The listing builds one solid part. Answer for the finished solid, in the listing's coordinates (mm). A direction names the side the tool comes from. Coordinates: 2 decimals unless noted, no trailing zeros. Write each loop counter-clockwise with the first axis right and the second up, starting at its lowest first coordinate (ties: lowest second). Pieces come first, ordered by that corner, then holes. Notation, with made-up numbers: M 27.25,-32 L 76.25,-32 A13 cw 76.25,-18 Z; hole C 7,83 d8. An arc over 180 degrees is marked long. Put each result on its own line as item: value. Start each with the question number.
Autodesk Fusion 360 part; units mm, degrees
sketch "Sketch1" plane through (0, 0, 0) normal (1, 0, 0) x (0, 1, 0)
  line L0 (-95, 52.5) -> (95, 52.5)
  line L1 (95, 52.5) -> (95, -52.5)
  line L2 (95, -52.5) -> (-95, -52.5)
  line L3 (-95, -52.5) -> (-95, 52.5)
  line L4 (95, 52.5) -> (-95, -52.5) construction
  line L5 (-95, 52.5) -> (95, -52.5) construction
  line L6 (92, -49.5) -> (-92, -49.5)
  line L7 (-92, -49.5) -> (-92, 49.5)
  line L8 (-92, 49.5) -> (92, 49.5)
  line L9 (92, 49.5) -> (92, -49.5)
  dimension "d1" = 190
  dimension "d2" = 105
  dimension "d5" = 3
extrude "Extrude1" add sketch "Sketch1" along normal blind 14 contours L0 L1 L2 L3 | L6 L7 L8 L9
extrude "Extrude2" cut sketch "Sketch1" along normal blind 10 contours L6 L7 L8 L9
fillet "Fillet1" radius 2.5 4 edges at (14, 0, -52.5) (14, 95, 0) (14, 0, 52.5) (14, -95, 0)
sketch "Sketch2" plane through (14, 0, 0) normal (1, 0, 0) x (0, 1, 0)
  line L0 (92.5, 50) -> (-92.5, 50)
  line L1 (-92.5, 50) -> (-92.5, -50)
  line L2 (-92.5, -50) -> (92.5, -50)
  line L3 (92.5, -50) -> (92.5, 50)
  circle A0 centre (0, 0) radius 7.5
  dimension "d10" = 15
extrude "Extrude3" cut sketch "Sketch2" against normal blind 40 contours A0
sketch "Sketch3" plane through (14, 0, 0) normal (1, 0, 0) x (0, 1, 0)
  circle A0 centre (0, 0) radius 7.5
  line L0 (92.5, 50) -> (-92.5, 50)
  line L1 (-92.5, 50) -> (-92.5, -50)
  line L2 (-92.5, -50) -> (92.5, -50)
  line L3 (92.5, -50) -> (92.5, 50)
  line L4 (-55, 27.5) -> (55, 27.5)
  line L5 (55, 27.5) -> (55, -27.5)
  line L6 (55, -27.5) -> (-55, -27.5)
  line L7 (-55, -27.5) -> (-55, 27.5)
  line L8 (55, 27.5) -> (-55, -27.5) construction
  line L9 (-55, 27.5) -> (55, -27.5) construction
  dimension "d13" = 110
  dimension "d14" = 55
hole "Hole1" at (14, 55, 27.5) at (14, -55, 27.5) at (14, -55, -27.5) at (14, 55, -27.5) direction (-1, 0, 0) diameter 1.371 depth 10 tip angle 118 counterbore diameter 3.5 counterbore depth 1.6
1) A cutting plane is placed at D-D on z = 23.5. Write down the section's boundary in (x, y).
2) Straight lines are drawn through the part: probe 1 along Z at (x, y) = (11.8, -55); probe 2 along Y at (x, z) = (10.55, 27.5); probe 3 along Y at (x, z) = (7.75, -37.5). For each, find the intervals that lie inside material, in ascending order.
3) A cutting plane is placed at C-C on y = -74. Write down the section's boundary in (x, z).
4) A cutting plane is placed at B-B on y = 0. Write down the section's boundary in (x, z).
5) Determine the mould class of faces 1 (the face through (14, -1, 12)), 2 (the face through (13.19, 56.06, 28.89)), 3 (the face through (10, -1, 12)), 4 (the face through (6, -95, -1)) for opening direction Y: +Y half, -Y half, draft (parallel to the pull), parting line (faces both ways), or undercut.
6) Given pin 1 Ø1.5 at (y, z) = (-35, 38.5) entering from -X; pin 2 Ø3 at (y, z) = (-55, -27.5) entering from +X; pin 3 Ø1.2 at (y, z) = (-55, -27.5) entering from +X, each flat-ended and moving along its own axis, determine where each tip first touches the part or whether it passes through.
7) For faces 5 (the face through (6, 1, -52.5)), 6 (the face through (5, -92, -1)), 7 (the face through (12.4, -54, -27)), determine the directions among +Z, -Z, +X, -X, +Y, -Y from which every point of the face is accessible in a straight line to the end or side of a thin tool.
8) A cutting plane is placed at A-A on z = 0. Write down the section's boundary in (x, y), then the cut area to 3 significant figures.
Answers follow:
1. outline: M 0,-95 L 11.5,-95 A2.5 ccw 14,-92.5 L 14,92.5 A2.5 ccw 11.5,95 L 0,95 L 0,92 L 10,92 L 10,-92 L 0,-92 Z
2. probe 1: z = -52.48 to -28.19, -26.81 to 26.81, 28.19 to 52.48
2. probe 2: y = -95 to -55.69, -54.31 to 54.31, 55.69 to 95
2. probe 3: y = -95 to -92, 92 to 95
3. outline: M 0,-52.5 L 11.5,-52.5 A2.5 ccw 14,-50 L 14,50 A2.5 ccw 11.5,52.5 L 0,52.5 L 0,49.5 L 10,49.5 L 10,-49.5 L 0,-49.5 Z
4. outline: M 0,-52.5 L 11.5,-52.5 A2.5 ccw 14,-50 L 14,-7.5 L 10,-7.5 L 10,-49.5 L 0,-49.5 Z; M 0,49.5 L 10,49.5 L 10,7.5 L 14,7.5 L 14,50 A2.5 ccw 11.5,52.5 L 0,52.5 Z
5. face 1: draft
5. face 2: undercut
5. face 3: undercut
5. face 4: -Y half
6. pin 1: stops at x = 10
6. pin 2: stops at x = 12.4
6. pin 3: passes through
7. face 5: -Z, +X, -X, +Y, -Y
7. face 6: -X
7. face 7: +X
8. outline: M 0,-95 L 11.5,-95 A2.5 ccw 14,-92.5 L 14,-7.5 L 10,-7.5 L 10,-92 L 0,-92 Z; M 0,92 L 10,92 L 10,7.5 L 14,7.5 L 14,92.5 A2.5 ccw 11.5,95 L 0,95 Z
8. area: 757 mm²
